```python
from build123d import *

# Parameters (mm, degrees)
F0_W     = 130.263165
F0_H     = 21.393939
F0_R     = 8
F1_DEPTH = 15
F2_R     = 10
F3_SIZE  = 2


with BuildPart() as f1:
    # F0 (on Front) → F1 (new body)
    with BuildSketch(Plane.XZ):
        with Locations((-1.332238, 27.719996)):
            Rectangle(F0_W, F0_H)
        with Locations((-51.963821, 27.916966)):
            Circle(F0_R, mode=Mode.SUBTRACT)
        with Locations((-25.963821, 27.916966)):
            Circle(F0_R, mode=Mode.SUBTRACT)
        with Locations((23.299344, 27.916966)):
            Circle(F0_R, mode=Mode.SUBTRACT)
        with Locations((49.299344, 27.916966)):
            Circle(F0_R, mode=Mode.SUBTRACT)
    extrude(amount=F1_DEPTH)

    # F2
    f2_edges = [f1.edges().sort_by_distance(p)[0] for p in [
        (63.799344, -7.5, 38.416966),
        (63.799344, -7.5, 17.023027),
        (-66.463821, -7.5, 38.416966),
        (-66.463821, -7.5, 17.023027),
    ]]
    fillet(f2_edges, radius=F2_R)

    # F3
    f3_edges = [f1.edges().sort_by_distance(p)[0] for p in [
        (-33.963821, -15, 27.916966),
        (15.299344, -15, 27.916966),
        (41.299344, -15, 27.916966),
        (-59.963821, -15, 27.916966),
    ]]
    chamfer(f3_edges, length=F3_SIZE)


solid = f1.part
```
Geometry: final body of the model. Coordinates: model frame, mm. Coordinates: 2 decimals unless noted, no trailing zeros. Order: outer loops, then holes, each group sorted by start corner. A loop starts at its lowest first (then second) coordinate and runs counter-clockwise, first axis right, second up. Notation, with made-up numbers: M -28.5,-26.75 L -18.5,-26.75 A16 cw -18.5,-17.75 Z; hole C -21,46.5 d10. An arc over 180 degrees is marked long. Answer in a Markdown table with one row per item. Add a question column.
Q1. Line query: L1, parallel to X at y = -4, z = 28.5; L2, parallel to X at y = -11.25, z = 26.25; L3, parallel to Z at x = -26.5, y = -10.5. Output: solid intervals per line, ascending.
Q2. Section query A-A on y = -8.25. Return the cut outline in (x, z), and give its area (3 significant figures).
Q3. Contact query for a flat-ended pin moving along its axis: P1, Ø8, axis at y = -13.5, z = 20.5, coming from the +X side. Output: stop coordinate, or through.
Q4. Mould query, pull axis X, two halves, no side actions, for faces 1 (the cylindrical face through (41.307, -6.409, 28.269)), 2 (the flat face through (-2, -15, 28)), 3 (the cylindrical face through (-63.61, -7.6, 20.03)). Classes: released by +X, released by -X, zero draft, split by the parting line, or undercut.
Q5. Section query B-B on z = 25.75. Count the separate pieces of the cut face and the enclosed holes in it, and give its area (3 significant figures).
Completed:
| question | item | result |
|---|---|---|
| 1 | L1 | x = -66.46 to -59.94, -43.99 to -33.94, -17.99 to 15.32, 31.28 to 41.32, 57.28 to 63.8 |
| 1 | L2 | x = -66.43 to -59.79, -44.14 to -33.79, -18.14 to 15.47, 31.12 to 41.47, 57.12 to 63.77 |
| 1 | L3 | z = 17.02 to 19.93, 35.9 to 38.42 |
| 2 | outline | M -66.46,27.02 A10 ccw -56.46,17.02 L 53.8,17.02 A10 ccw 63.8,27.02 L 63.8,28.42 A10 ccw 53.8,38.42 L -56.46,38.42 A10 ccw -66.46,28.42 Z; hole C -51.96,27.92 d16; hole C -25.96,27.92 d16; hole C 23.3,27.92 d16; hole C 49.3,27.92 d16 |
| 2 | area | 1,900 mm2 |
| 3 | P1 | stops at x = 63.48 |
| 4 | face 1 | undercut |
| 4 | face 2 | zero draft |
| 4 | face 3 | released by -X |
| 5 | separate pieces | 5 |
| 5 | enclosed holes | 0 |
| 5 | area | 1,010 mm2 |
